```python
from build123d import *

# Parameters (mm, degrees)
SKETCH1_R           = 3.175
BOSS_EXTRUDE1_DEPTH = 0.79375
SKETCH2_R           = 2.38125
BOSS_EXTRUDE2_DEPTH = 3.175
SKETCH3_R           = 1.5875
BOSS_EXTRUDE3_DEPTH = 3.175
FILLET1_R           = 0.254


with BuildPart() as part:
    # Sketch1 → Boss-Extrude1 (new body)
    with BuildSketch(Plane(origin=(0, 0, 0), x_dir=(1, 0, 0), z_dir=(0, 1, 0))):
        with Locations(Location((0, 0, 0), (0, 0, 270))):
            Circle(SKETCH1_R)
    extrude(amount=BOSS_EXTRUDE1_DEPTH)

    # Sketch2 → Boss-Extrude2 (add)
    with BuildSketch(Plane(origin=(0, 0.79375, 0), x_dir=(1, 0, 0), z_dir=(0, 1, 0))):
        with Locations(Location((0, 0, 0), (0, 0, 270))):
            Circle(SKETCH2_R)
    extrude(amount=BOSS_EXTRUDE2_DEPTH)

    # Sketch3 → Boss-Extrude3 (add)
    with BuildSketch(Plane(origin=(0, 3.96875, 0), x_dir=(1, 0, 0), z_dir=(0, 1, 0))):
        with Locations(Location((0, 0, 0), (0, 0, 270))):
            Circle(SKETCH3_R)
    extrude(amount=BOSS_EXTRUDE3_DEPTH)

    # Fillet1
    fillet1_edges = [part.edges().sort_by_distance(p)[0] for p in [
        (0, 0, -3.175),
    ]]
    fillet(fillet1_edges, radius=FILLET1_R)


solid = part.part
```
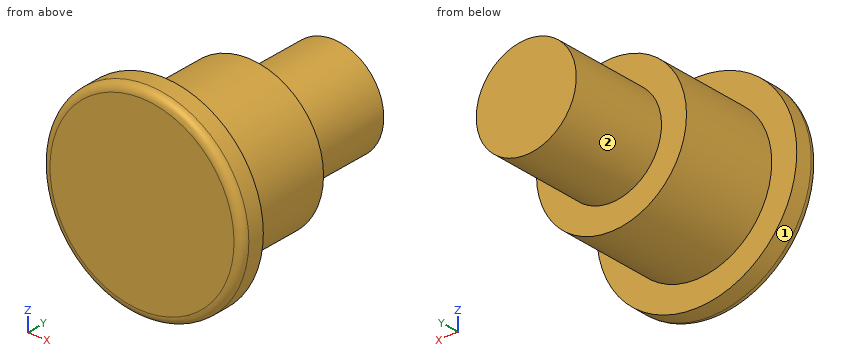
Design review of the part built by this model. Coordinates are the model's own, in mm. Face numbers are marked on the shaded views. A direction names the side the tool comes from. Coordinates: 2 decimals unless noted, no trailing zeros. Order: outer loops, then holes, each group sorted by start corner. A loop starts at its lowest first (then second) coordinate and runs counter-clockwise, first axis right, second up.
1) Take a section at D-D, the plane y = 5.5. Give the boundary of the cut face in (x, z) (1 decimal).
2) Clearance check with flat-ended pins moving along their axes: pin 1 (3 mm diameter, centred on y = 2, z = 1.5, fed in from -X); pin 2 (2 mm diameter, centred on x = -2.5, y = 2, fed in from +Z). State where each tip first meets the part, or that it passes through.
3) Wall thickness on line 1 along Y through (x, z) = (-2.25, 0.25); line 2 along Y through (x, z) = (2, -1.5); line 3 along Z through (x, y) = (-1.5, 1): over which ranges is each line inside the solid? List them lowest first.
4) Take a section at C-C, the plane y = 2.5. Give the boundary of the cut face in (x, z), and give its area (3 significant figures).
5) For the marked faces 1 and 2, list the 3-axis set-ups (+Z, -Z, +X, -X, +Y, -Y) from which the entire face can be reached by the end or side of a thin tool; tool diameter is ignored.
Returned:
1. outline: circle Ø3.2 at (0, 0)
2. pin 1: stops at x = -3.12
2. pin 2: stops at z = 1.85
3. line 1: y = 0 to 3.97
3. line 2: y = 0 to 0.79
3. line 3: z = -1.85 to 1.85
4. outline: circle Ø4.76 at (0, 0)
4. area: 17.8 mm2
5. face 1: +Y, -Y
5. face 2: +Y
